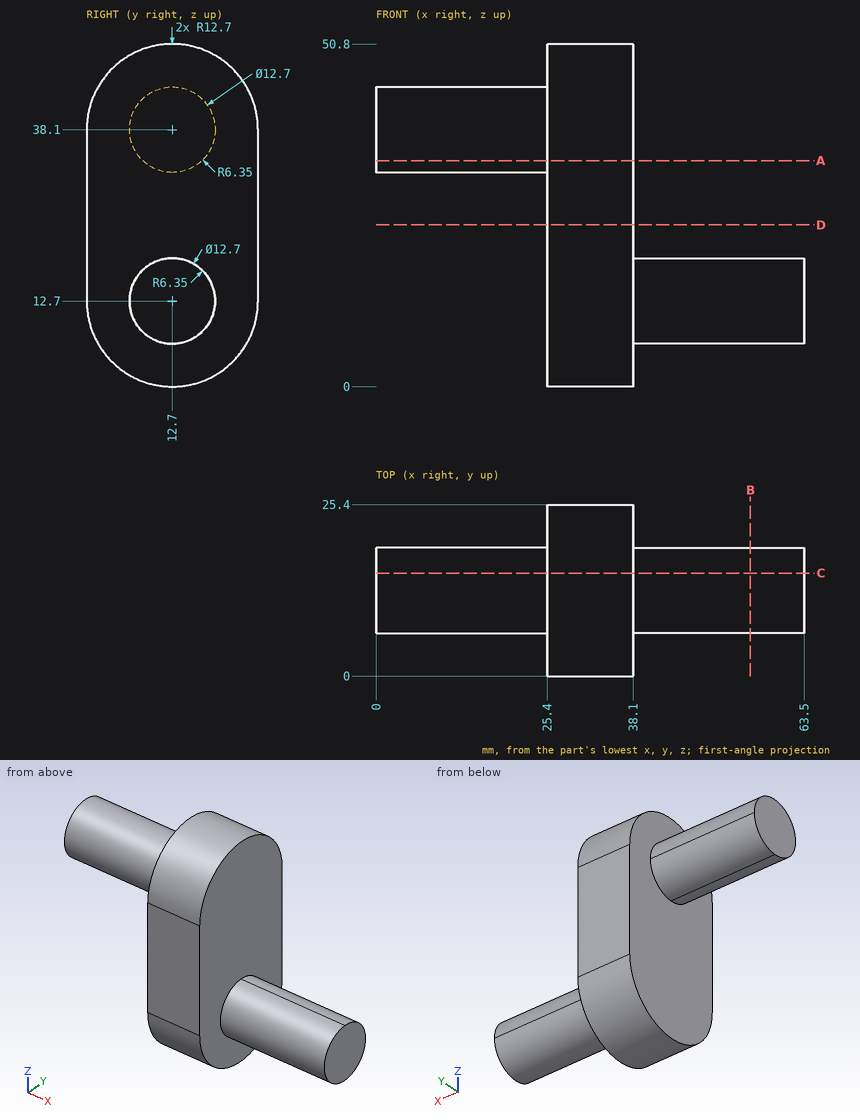
Input: dimensioned drawing with shaded views. Units: mm. Origin: part minimum x, y, z. Round coordinates to 2 decimals unless told otherwise and drop trailing zeros. Loops run counter-clockwise (first coordinate to the right, second up) from the corner with the lowest first, then second, coordinate; pieces in that order, holes last. Notation, with made-up numbers: (28, 0.25) -> (75, 0.25) arc R26 ccw to (75, 31.25) -> close; hole circle Ø9 at (9, 68.5). An arc over 180 degrees is marked (long way). One line per item, written item: value.
(1) Section A-A (z = 33.5). Return the cut outline in (x, y), plus the area to 3 significant figures.
Geometry check:
outline: (0, 8.32) -> (25.4, 8.32) -> (25.4, 0) -> (38.1, 0) -> (38.1, 25.4) -> (25.4, 25.4) -> (25.4, 17.08) -> (0, 17.08) -> close
area: 545 mm2
(2) Section D-D (z = 24). Return the cut outline in (x, y), plus the area to 3 significant figures.
Geometry check:
outline: (25.4, 0) -> (38.1, 0) -> (38.1, 25.4) -> (25.4, 25.4) -> close
area: 323 mm2
(3) Pin query (flat end, axial travel): pin 1 (8 mm diameter, centred on y = 8.5, z = 18.5, fed in from +X); pin 2 (1.5 mm diameter, centred on y = 6.5, z = 35.5, fed in from +X); pin 3 (1.5 mm diameter, centred on x = 53, y = 18.5, fed in from +Z); pin 4 (6 mm diameter, centred on x = 14.5, y = 6.5, fed in from -Z). Return the tip coordinate at first contact, or that it passes through.
Geometry check:
pin 1: x = 63.5
pin 2: x = 38.1
pin 3: z = 16.55
pin 4: z = 32.62
(4) Material intervals for line 1 (X direction, y = 19.5, z = 10.5); line 2 (X direction, y = 15.5, z = 43); line 3 (Y direction, x = 22, z = 43), sorted ascending. Write a range as [from, to].
Geometry check:
line 1: [25.4, 38.1]
line 2: [0, 38.1]
line 3: [8.66, 16.74]
(5) Section C-C (y = 15.25). Return the cut outline in (x, z), plus the area to 3 significant figures.
Geometry check:
outline: (0, 32.28) -> (25.4, 32.28) -> (25.4, 0.26) -> (38.1, 0.26) -> (38.1, 6.88) -> (63.5, 6.88) -> (63.5, 18.52) -> (38.1, 18.52) -> (38.1, 50.54) -> (25.4, 50.54) -> (25.4, 43.92) -> (0, 43.92) -> close
area: 1,230 mm2
(6) Section B-B (x = 55.5). Return the cut outline in (y, z).
Geometry check:
outline: circle Ø12.7 at (12.7, 12.7)
